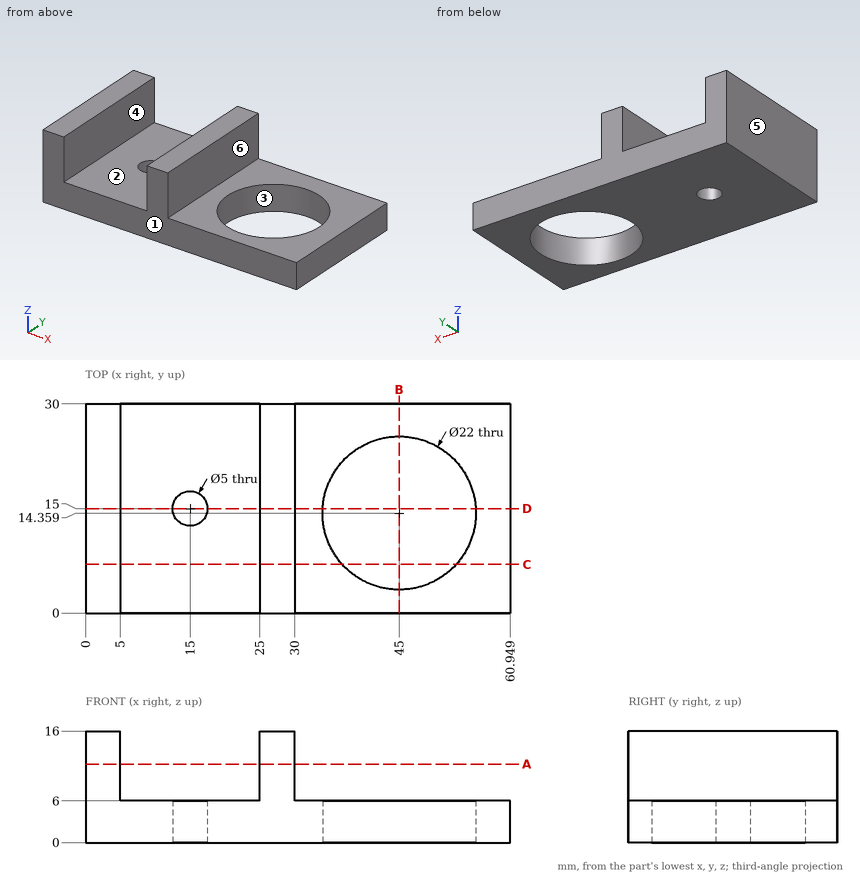
The drawing under review shows one solid part. Ordinate dimensions are in mm from its lowest x, y, z. A direction names the side the tool comes from. Round coordinates to 2 decimals unless told otherwise and drop trailing zeros. Write each loop counter-clockwise with the first axis right and the second up, starting at its lowest first coordinate (ties: lowest second). Pieces come first, ordered by that corner, then holes. Notation, with made-up numbers: (25.25, 67) -> (54.25, 67) arc R34 ccw to (54.25, 105) -> close; hole circle Ø2 at (-3, 39). An arc over 180 degrees is marked (long way). Put each result on its own line as item: value.
Q1. Consider section C-C on y = 7. State the section outline as (x, z) points (1 decimal).
Determined:
outline: (0, 0) -> (36.8, 0) -> (36.8, 6) -> (30, 6) -> (30, 16) -> (25, 16) -> (25, 6) -> (5, 6) -> (5, 16) -> (0, 16) -> close; (53.2, 0) -> (60.9, 0) -> (60.9, 6) -> (53.2, 6) -> close
Q2. Machinability: for the marked faces 4, 5 and 6, which of the approach directions +Z, -Z, +X, -X, +Y, -Y give a long, thin tool a straight path to every point of the face, cutting with its end or side? Answer none if there is none.
Determined:
face 4: +Z, +Y, -Y
face 5: +Z, -Z, -X, +Y, -Y
face 6: +Z, +X, +Y, -Y
Q3. To check wall thickness, follow L1, parallel to X at y = 24.5, z = 12.75; L2, parallel to Y at x = 15, z = 1.6; L3, parallel to Y at x = 45, z = 2.15. State the ranges of each line that lie inside material, in increasing order. Write a range as [from, to].
Determined:
L1: x = [0, 5], [25, 30]
L2: y = [0, 12.5], [17.5, 30]
L3: y = [0, 3.36], [25.36, 30]
Q4. Consider section D-D on y = 15. State the section outline as (x, z) points, and give its area (3 significant figures).
Determined:
outline: (0, 0) -> (12.5, 0) -> (12.5, 6) -> (5, 6) -> (5, 16) -> (0, 16) -> close; (17.5, 0) -> (34.02, 0) -> (34.02, 6) -> (30, 6) -> (30, 16) -> (25, 16) -> (25, 6) -> (17.5, 6) -> close; (55.98, 0) -> (60.95, 0) -> (60.95, 6) -> (55.98, 6) -> close
area: 304 mm^2
Q5. Consider section B-B on x = 45. State the section outline as (y, z) points, and give its area (3 significant figures).
Determined:
outline: (0, 0) -> (3.36, 0) -> (3.36, 6) -> (0, 6) -> close; (25.36, 0) -> (30, 0) -> (30, 6) -> (25.36, 6) -> close
area: 48.0 mm^2
Q6. The part is to be moulded in two halves that separate along Y. For the marked faces 1, 2 and 3, say which applies: released by +Y, released by -Y, zero draft, split by the parting line, or undercut.
Determined:
face 1: released by -Y
face 2: zero draft
face 3: undercut
Q7. Consider section A-A on z = 11.25. State the section outline as (x, y) points.
Determined:
outline: (0, 0) -> (5, 0) -> (5, 30) -> (0, 30) -> close; (25, 0) -> (30, 0) -> (30, 30) -> (25, 30) -> close
Q8. Clearance check with flat-ended pins moving along their axes: pin 1 Ø2 at (x, y) = (16.5, 14.5) entering from -Z; pin 2 Ø1.5 at (x, y) = (15, 9.5) entering from +Z; pin 3 Ø5 at (y, z) = (10.5, 11) entering from +X. State where each tip first meets the part, or that it passes through.
Determined:
pin 1: stops at z = 0
pin 2: stops at z = 6
pin 3: stops at x = 30
